```python
from build123d import *

# Parameters (mm, degrees)
SKETCH_1_W      = 19
SKETCH_1_H      = 2.5
EXTRUDE_1_DEPTH = 2
EXTRUDE_2_DEPTH = 2


with BuildPart() as part:
    # 草图1 → 凸台-拉伸1 (new body)
    # profile 1 of 2: a face of its own
    with BuildSketch(Plane.XY):
        with BuildLine():
            Line((-9.5, 55.5), (-9.5, 2.5))
            Line((-9.5, 2.5), (9.5, 2.5))
            Line((9.5, 2.5), (9.5, 55.5))
            ThreePointArc((9.5, 55.5), (0, 65), (-9.5, 55.5))
        make_face()
        with BuildLine():
            ThreePointArc((-2.5, 53), (0, 55.5), (2.5, 53))
            Line((2.5, 53), (2.5, 10))
            ThreePointArc((2.5, 10), (0, 7.5), (-2.5, 10))
            Line((-2.5, 10), (-2.5, 53))
        make_face(mode=Mode.SUBTRACT)
    # profile 2 of 2: a face of its own
    with BuildSketch(Plane.XY):
        with Locations((0, 1.25)):
            Rectangle(SKETCH_1_W, SKETCH_1_H)
    extrude(amount=EXTRUDE_1_DEPTH)

    # 草图2 → 凸台-拉伸2 (add)
    with BuildSketch(Plane(origin=(0, 0, 0), x_dir=(1, 0, 0), z_dir=(0, 1, 0))):
        with BuildLine():
            Line((-9.5, -2), (9.5, -2))
            Line((9.5, -2), (9.5, 53.5))
            ThreePointArc((9.5, 53.5), (0, 63), (-9.5, 53.5))
            Line((-9.5, 53.5), (-9.5, -2))
        make_face()
        with BuildLine():
            Line((-2.5, 8), (-2.5, 51))
            ThreePointArc((-2.5, 51), (0, 53.5), (2.5, 51))
            Line((2.5, 51), (2.5, 8))
            ThreePointArc((2.5, 8), (0, 5.5), (-2.5, 8))
        make_face(mode=Mode.SUBTRACT)
    extrude(amount=EXTRUDE_2_DEPTH)


solid = part.part
```
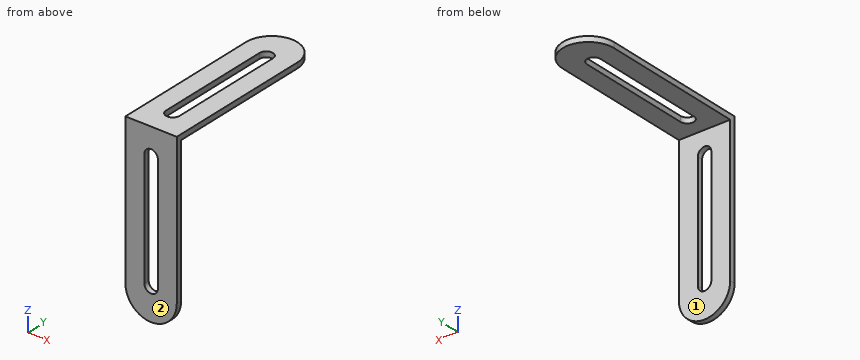
Read the model definition and answer for the solid it produces. Units are mm, in the model's axes. Face numbers are marked on the shaded views. A direction names the side the tool comes from. Round coordinates to 2 decimals unless told otherwise and drop trailing zeros. Write each loop counter-clockwise with the first axis right and the second up, starting at its lowest first coordinate (ties: lowest second). Pieces come first, ordered by that corner, then holes. Notation, with made-up numbers: (-6.75, 16) - (38.25, 16) arc R28 ccw to (38.25, 54) - close; hole circle Ø11 at (41.5, 84). An arc over 180 degrees is marked (long way). One line per item, written item: value.
Q1. Find section A-A (x = 0). Determine the outline of the cut face in (y, z).
The answers:
outline: (0, -63) - (2, -63) - (2, -53.5) - (0, -53.5) - close; (0, -5.5) - (2, -5.5) - (2, 0) - (7.5, 0) - (7.5, 2) - (0, 2) - close; (55.5, 0) - (65, 0) - (65, 2) - (55.5, 2) - close
Q2. Each of these flat-tipped pins is pushed along its axis until it touches: P1, Ø9.5, axis at x = 0, y = 32, coming from the -Z side; P2, Ø4, axis at x = -3.5, z = -27, coming from the +Y side. Where does it stop, or does it pass through?
The answers:
P1: stops at z = 0
P2: stops at y = 2
Q3. A straight line is drawn through the part: line 1 (Y direction, x = 3, z = -43). Find the intervals that lie inside material, in ascending order. Write a range as from..to.
The answers:
line 1: y = 0..2
Q4. Which of the six approach directions +Z, -Z, +X, -X, +Y, -Y give full straight-line access (tool end or side, diameter ignored) to the marked faces 1 and 2?
The answers:
face 1: -Z, +X, -X, +Y
face 2: +Z, -Z, +X, -X, -Y
Q5. Find section D-D (x = -7.5). Determine the outline of the cut face in (y, z), and give its area (3 significant figures).
The answers:
outline: (0, -59.33) - (2, -59.33) - (2, 0) - (61.33, 0) - (61.33, 2) - (0, 2) - close
area: 241 mm2
Q6. Find section B-B (y = 28). Determine the outline of the cut face in (x, z).
The answers:
outline: (-9.5, 0) - (-2.5, 0) - (-2.5, 2) - (-9.5, 2) - close; (2.5, 0) - (9.5, 0) - (9.5, 2) - (2.5, 2) - close
